CAD build for the part. Positions are in the model's coordinates, mm. Coordinates: 2 decimals unless noted, no trailing zeros. Loops run counter-clockwise (first coordinate to the right, second up) from the corner with the lowest first, then second, coordinate; pieces in that order, holes last. Notation, with made-up numbers: M 56,79.5 L 88,79.5 A10 cw 88,97.5 Z; hole C -8.75,-36 d9. An arc over 180 degrees is marked long. Answer as a JSON object with one key per item and string values. Group by question number.
```python
from build123d import *

# Parameters (mm, degrees)
BOSS_EXTRUDE1_DEPTH = 10
SKETCH2_R           = 1.5
CUT_EXTRUDE1_DEPTH  = 15
SKETCH3_R           = 1.5
CUT_EXTRUDE2_DEPTH  = 15


with BuildPart() as part:
    # Sketch1 → Boss-Extrude1 (new body)
    with BuildSketch(Plane(origin=(0, 0, 0), x_dir=(1, 0, 0), z_dir=(0, 1, 0))):
        Polygon((-125, 200), (-125, 125), (-115, 125), (-115, 75), (-125, 75), (-125, 25), (-100, 0), (100, 0), (125, 25), (125, 75), (115, 75), (115, 125), (125, 125), (125, 200), (75, 260), (25, 260), (25, 250), (-25, 250), (-25, 260), (-75, 260), align=None)
    extrude(amount=BOSS_EXTRUDE1_DEPTH)

    # Sketch2 → Cut-Extrude1 (cut)
    with BuildSketch(Plane.ZY.offset(115)):
        with Locations((-113, 5)):
            Circle(SKETCH2_R)
        with Locations((-87, 5)):
            Circle(SKETCH2_R)
    cut_extrude1 = extrude(amount=-CUT_EXTRUDE1_DEPTH, mode=Mode.SUBTRACT)

    # Mirror1: Cut-Extrude1 across plane
    add(cut_extrude1.mirror(Plane(origin=(0, 0, 0), x_dir=(0, 0, 1), z_dir=(1, 0, 0))), mode=Mode.SUBTRACT)

    # Sketch3 → Cut-Extrude2 (cut)
    with BuildSketch(Plane(origin=(0, 0, -250), x_dir=(-1, 0, 0), z_dir=(0, 0, -1))):
        with Locations((-13, 5)):
            Circle(SKETCH3_R)
        with Locations((13, 5)):
            Circle(SKETCH3_R)
    extrude(amount=-CUT_EXTRUDE2_DEPTH, mode=Mode.SUBTRACT)


solid = part.part
```
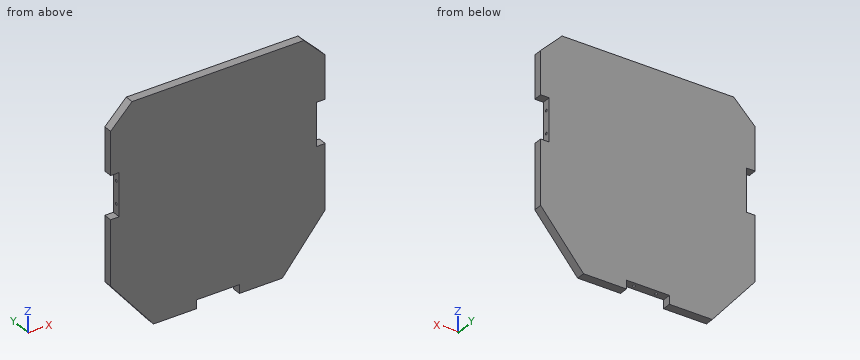
Item 1: Pin check, flat tips, straight feed: pin 1 (1.5 mm diameter, centred on y = 4.5, z = -222, fed in from -X); pin 2 (2.5 mm diameter, centred on y = 5, z = -87, fed in from +X); pin 3 (3 mm diameter, centred on y = 2.5, z = -95, fed in from +X). Stop position of each tip, or through.
Item 2: Slice it at C-C, the plane z = -78. Write the cut outline in (x, y), then the cut area to 3 significant figures.
Item 3: Slice it at B-B, the plane z = -238. Write the cut outline in (x, y).
Item 4: Drill centre lines: L1, parallel to Y at x = -105, z = -87; L2, parallel to Z at x = -2.5, y = 7.25; L3, parallel to Z at x = 86, y = 3.25. Where is each one in solid material? Low to high. Write a range as from..to.
Item 5: Slice it at A-A, the plane x = 104. Write the cut outline in (y, z).
Computed:
{
 "1": {"pin 1": "x = -107.29", "pin 2": "x = 100", "pin 3": "x = 115"},
 "2": {"outline": "M -115,0 L 115,0 L 115,10 L -115,10 Z", "area": "2,300 mm2"},
 "3": {"outline": "M -93.33,0 L 93.33,0 L 93.33,10 L -93.33,10 Z; hole C -13,5 d3; hole C 13,5 d3"},
 "4": {"L1": "0..3.5, 6.5..10", "L2": "-250..0", "L3": "-246.8..0"},
 "5": {"outline": "M 0,-225.2 L 10,-225.2 L 10,-4 L 0,-4 Z; hole C 5,-113 d3; hole C 5,-87 d3"}
}
